Part model, mm, in its own coordinate system. A direction names the side the tool comes from. Coordinates: 2 decimals unless noted, no trailing zeros. Order: outer loops, then holes, each group sorted by start corner. A loop starts at its lowest first (then second) coordinate and runs counter-clockwise, first axis right, second up. Notation, with made-up numbers: (39.25, 60.5) - (47.25, 60.5) arc R26 ccw to (47.25, 88.5) - close; hole circle Ø6 at (-24, 17.25). An arc over 180 degrees is marked (long way). Use a Markdown table: item, result. Add a question column.
1) Two-plate mould, pull along Z, no slides. Class faces 6 (the face through (9, 21, 0)), 7 (the face through (-11.5, 21.2, 0)), 8 (the face through (-4.1, 17, 7)): +Z half, -Z half, draft (parallel to the pull), parting line (faces both ways), or undercut.
2) Saw through at C-C on x = 10. List the corners of the cut face in (y, z), then the cut area to 3 significant figures.
3) Saw through at D-D on z = 2.5. List the corners of the cut face in (x, y).
4) Tool access for faces 1 (the face through (-7.75, 0.49, -0.03)), 2 (the face through (-8.537, -2.916, -0.056)), 3 (the face through (-7.5, 0.5, 3)), 4 (the face through (-3.417, 1.986, -0.759)), 5 (the face through (-8.764, 21.186, 3.279)): list every direction of +Z, -Z, +X, -X, +Y, -Y with a clear straight run to the whole face (end or side of a thin tool).
5) Wall check: L1, parallel to X at y = 20.85, z = 0; L2, parallel to Y at x = 7, z = 1.75; L3, parallel to X at y = 13.5, z = 0. Give the ranges that are in metal, low to high. Write a range as [from, to].
6) Saw through at A-A on y = 10. List the corners of the cut face in (x, z).
7) Saw through at B-B on x = 0. List the corners of the cut face in (y, z).
8) Drop flat-ended pins along their axis: P1, Ø3, axis at y = -5.5, z = 2, coming from the +X side; P2, Ø9.5, axis at x = -2.5, y = 4.5, coming from the -Z side; P3, Ø1.2, axis at x = -6, z = 0, coming from the +Y side; P4, Ø9, axis at y = 10, z = -2, coming from the -X side. Give the stop position or say it passes through.
```python
from build123d import *
from build123d.topology import SkipClean

# Parameters (mm, degrees)
SKETCH_2_W                = 19
SKETCH_2_H                = 8
EXTRUDE_1_DEPTH           = 9
SKETCH_4_R                = 8.5
EXTRUDE_2_DEPTH           = 22.2
CUT_EXTRUDE_5_REACH       = 27.6
SKETCH_5_2_R              = 7.75
EXTRUDE_START             = -2
SKETCH_9_R                = 1
EXTRUDE_4_DEPTH           = 2
SKETCH_5_R                = 7.75
CUT_EXTRUDE_8_DEPTH       = 27.407196
SKETCH_11_W               = 15.2
SKETCH_11_H               = 8
CUT_EXTRUDE_11_DEPTH      = 4
SKETCH_12_W               = 8.2
SKETCH_12_H               = 22.2
CUT_EXTRUDE_12_DEPTH      = 27.407196
SKETCH_13_W               = 11.493961
SKETCH_13_H               = 8
CUT_EXTRUDE_13_DEPTH      = 27.407196
EXTRUDE_6_DEPTH           = 3
EXTRUDE_7_DEPTH           = 15
SKETCH_16_R               = 1
CUT_EXTRUDE_14_DEPTH      = 30.848618
SKETCH_17_R               = 8.5
SKETCH_17_R_2             = 3.5
EXTRUDE_8_DEPTH           = 2
CUT_EXTRUDE_15_DEPTH      = 27.407196
CUT_EXTRUDE_15_DEPTH_BACK = 27.407196
CUT_EXTRUDE_17_DEPTH      = 1


with BuildPart() as part:
    # Sketch 2 → Extrude 1 (new body)
    with BuildSketch(Plane(origin=(0, 0, 0), x_dir=(1, 0, 0), z_dir=(0, 1, 0))):
        Rectangle(SKETCH_2_W, SKETCH_2_H)
    extrude(amount=-EXTRUDE_1_DEPTH)

    # Sketch 4 → Extrude 2 (add)
    with BuildSketch(Plane(origin=(0, 0, 0), x_dir=(1, 0, 0), z_dir=(0, 1, 0))):
        with Locations(Location((0, 0, 0), (0, 0, 28.072487))):
            Circle(SKETCH_4_R)
    extrude(amount=EXTRUDE_2_DEPTH)

    # Sketch 5_2 → Cut-Extrude 5 (cut, up to next)
    with BuildSketch(Plane(origin=(0, 0, 0), x_dir=(1, 0, 0), z_dir=(0, 1, 0)), mode=Mode.PRIVATE) as cut_extrude_5_sk1:
        with Locations(Location((0, 0, 0), (0, 0, 31.072951))):
            Circle(SKETCH_5_2_R)
    cut_extrude_5_tool1 = extrude(cut_extrude_5_sk1.sketch, amount=CUT_EXTRUDE_5_REACH, mode=Mode.PRIVATE) & part.part
    add(cut_extrude_5_tool1.solids().sort_by_distance((0, 0, 0))[0], mode=Mode.SUBTRACT)

    # Sketch 9 → Extrude 4 (add)
    with SkipClean():  # the faces are left unmerged after this step: merging them gives an invalid solid
        with BuildSketch(Plane(origin=(0, 22.2, 0), x_dir=(1, 0, 0), z_dir=(0, 1, 0)).offset(EXTRUDE_START)):
            with BuildLine():
                Line((-11.05, 1.071214), (-5.95, 6.070214))
                ThreePointArc((-5.95, 6.070214), (0, 8.5), (5.95, 6.070214))
                Line((5.95, 6.070214), (11.05, 1.071214))
                ThreePointArc((11.05, 1.071214), (11.49999, -0.005522), (11.042085, -1.078916))
                Line((11.042085, -1.078916), (6.548688, -5.418919))
                ThreePointArc((6.548688, -5.418919), (0, -8.5), (-6.548688, -5.418919))
                Line((-6.548688, -5.418919), (-11.042085, -1.078916))
                ThreePointArc((-11.042085, -1.078916), (-11.49999, -0.005522), (-11.05, 1.071214))
            make_face()
            with Locations(Location((-10, 0, 0), (0, 0, 270))):
                Circle(SKETCH_9_R, mode=Mode.SUBTRACT)
            with Locations(Location((10, 0, 0), (0, 0, 90))):
                Circle(SKETCH_9_R, mode=Mode.SUBTRACT)
        extrude(amount=EXTRUDE_4_DEPTH)

    # Sketch 5 → Cut-Extrude 8 (cut, through all)
    with SkipClean():  # the faces are left unmerged after this step: merging them gives an invalid solid
        with BuildSketch(Plane(origin=(0, 0, 0), x_dir=(1, 0, 0), z_dir=(0, 1, 0))):
            with Locations(Location((0, 0, 0), (0, 0, 31.072951))):
                Circle(SKETCH_5_R)
        extrude(amount=CUT_EXTRUDE_8_DEPTH, mode=Mode.SUBTRACT)

    # Sketch 11 → Cut-Extrude 11 (cut)
    with SkipClean():  # the faces are left unmerged after this step: merging them gives an invalid solid
        with BuildSketch(Plane(origin=(0, 0, 0), x_dir=(1, 0, 0), z_dir=(0, 1, 0))):
            Rectangle(SKETCH_11_W, SKETCH_11_H)
        extrude(amount=-CUT_EXTRUDE_11_DEPTH, mode=Mode.SUBTRACT)

    # Sketch 12 → Cut-Extrude 12 (cut, through all)
    with SkipClean():  # the faces are left unmerged after this step: merging them gives an invalid solid
        with BuildSketch(Plane.XY):
            with Locations((0, 11.1)):
                Rectangle(SKETCH_12_W, SKETCH_12_H)
        extrude(amount=CUT_EXTRUDE_12_DEPTH, mode=Mode.SUBTRACT)

    # Sketch 13 → Cut-Extrude 13 (cut, through all)
    with SkipClean():  # the faces are left unmerged after this step: merging them gives an invalid solid
        with BuildSketch(Plane(origin=(0, 0, 0), x_dir=(0, 0, -1), z_dir=(1, 0, 0))):
            with Locations((-1.698824, 7)):
                Rectangle(SKETCH_13_W, SKETCH_13_H)
        extrude(amount=-CUT_EXTRUDE_13_DEPTH, mode=Mode.SUBTRACT)

    # Sketch 14 → Extrude 6 (add)
    with BuildSketch(Plane(origin=(0, 0, 0), x_dir=(1, 0, 0), z_dir=(0, 1, 0))):
        with BuildLine():
            Line((-7.6, 3.806573), (-7.6, 4))
            Line((-7.6, 4), (-9.5, 4))
            Line((-9.5, 4), (-9.5, -4))
            Line((-9.5, -4), (-7.6, -4))
            Line((-7.6, -4), (-7.6, -3.806573))
            ThreePointArc((-7.6, -3.806573), (-8.5, 0), (-7.6, 3.806573))
        make_face()
    extrude(amount=EXTRUDE_6_DEPTH)

    # Sketch 15 → Extrude 7 (add)
    with SkipClean():  # the faces are left unmerged after this step: merging them gives an invalid solid
        with BuildSketch(Plane(origin=(0, 0, 0), x_dir=(1, 0, 0), z_dir=(0, 1, 0))):
            with BuildLine():
                Line((7.6, -3.806573), (7.6, -4))
                Line((7.6, -4), (9.5, -4))
                Line((9.5, -4), (9.5, 4))
                Line((9.5, 4), (7.6, 4))
                Line((7.6, 4), (7.6, 3.806573))
                ThreePointArc((7.6, 3.806573), (8.5, 0), (7.6, -3.806573))
            make_face()
        extrude(amount=EXTRUDE_7_DEPTH)

    # Sketch 16 → Cut-Extrude 14 (cut, through all)
    with SkipClean():  # the faces are left unmerged after this step: merging them gives an invalid solid
        with BuildSketch(Plane(origin=(0, -4, 0), x_dir=(1, 0, 0), z_dir=(0, 1, 0))):
            with Locations(Location((-6, 0, 0), (0, 0, 270))):
                Circle(SKETCH_16_R)
            with Locations(Location((6, 0, 0), (0, 0, 90))):
                Circle(SKETCH_16_R)
        extrude(amount=-CUT_EXTRUDE_14_DEPTH, mode=Mode.SUBTRACT)

    # Sketch 17 → Extrude 8 (add)
    with BuildSketch(Plane(origin=(0, 3, 0), x_dir=(1, 0, 0), z_dir=(0, 1, 0)).offset(EXTRUDE_START)):
        Circle(SKETCH_17_R)
        with Locations(Location((0, 0, 0), (0, 0, 270))):
            Circle(SKETCH_17_R_2, mode=Mode.SUBTRACT)
    extrude(amount=EXTRUDE_8_DEPTH)

    # Sketch 18 → Cut-Extrude 15 (cut, two sides: drawn at the far end of the back side and taken through both)
    with BuildSketch(Plane.XY.offset(-CUT_EXTRUDE_15_DEPTH_BACK)):
        Polygon((-7.6, 3), (-9.5, -9), (-9.5, 3), align=None)
    extrude(amount=CUT_EXTRUDE_15_DEPTH + CUT_EXTRUDE_15_DEPTH_BACK, mode=Mode.SUBTRACT)

    # Sketch 19 → Cut-Extrude 17 (cut)
    with BuildSketch(Plane(origin=(0, 0, 0), x_dir=(1, 0, 0), z_dir=(0, 1, 0))):
        with BuildLine():
            Line((-7.5, -4), (-7.5, 4))
            ThreePointArc((-7.5, 4), (8.5, 0), (-7.5, -4))
        make_face()
    extrude(amount=CUT_EXTRUDE_17_DEPTH, mode=Mode.SUBTRACT)


solid = part.part
```
Results are:
| question | item | result |
|---|---|---|
| 1 | face 6 | undercut |
| 1 | face 7 | parting line |
| 1 | face 8 | draft |
| 2 | outline | (20.2, -2.1) - (22.2, -2.1) - (22.2, -1) - (20.2, -1) - close; (20.2, 1) - (22.2, 1) - (22.2, 2.09) - (20.2, 2.09) - close |
| 2 | area | 4.37 mm2 |
| 3 | outline | (-9.57, 20.2) - (-8.12, 20.2) - (-8.12, 11) - (-7.34, 11) - (-7.34, 22.2) - (-9.57, 22.2) - close; (-9.5, -9) - (9.5, -9) - (9.5, 15) - (8.12, 15) - (8.12, 20.2) - (9.57, 20.2) - (9.57, 22.2) - (7.34, 22.2) - (7.34, 3) - (2.45, 3) - (2.45, 1) - (8.12, 1) - (8.12, 0) - (7.6, 0) - (7.6, -4) - (-7.6, -4) - (-7.6, 0) - (-7.5, 0) - (-7.5, 1) - (-2.45, 1) - (-2.45, 3) - (-7.6, 3) - close |
| 4 | face 1 | none |
| 4 | face 2 | +Z, -Z, -X |
| 4 | face 3 | +Z, -Z |
| 4 | face 4 | +Y |
| 4 | face 5 | +Z, -X, +Y |
| 5 | L1 | [-11.5, -11], [-9, -7.75], [7.75, 9], [11, 11.5] |
| 5 | L2 | [-9, -4], [1, 3] |
| 5 | L3 | [-8.5, -7.75], [7.75, 9.5] |
| 6 | outline | (-7.47, -4.05) arc R8.5 ccw to (7.6, -3.81) - (7.6, -4) - (9.5, -4) - (9.5, 4) - (7.6, 4) - (7.6, 3.81) arc R8.5 ccw to (4.1, 7.45) - (4.1, 6.58) arc R7.75 cw (long way) to (-6.61, -4.05) - close |
| 7 | outline | (-9, -4) - (-4, -4) - (-4, 4) - (-9, 4) - close; (1, -8.5) - (22.2, -8.5) - (22.2, -7.75) - (3, -7.75) - (3, -3.5) - (1, -3.5) - close; (1, 3.5) - (3, 3.5) - (3, 8.5) - (1, 8.5) - close |
| 8 | P1 | x = 9.5 |
| 8 | P2 | z = -8.5 |
| 8 | P3 | y = 3 |
| 8 | P4 | x = -8.5 |
